Part print with two shaded views. Sizes in mm from the minimum x, y, z corner. Give positions to 0.01 mm unless a question says otherwise; leave off trailing zeros. Write each loop counter-clockwise with the first axis right and the second up, starting at its lowest first coordinate (ties: lowest second). Pieces come first, ordered by that corner, then holes.
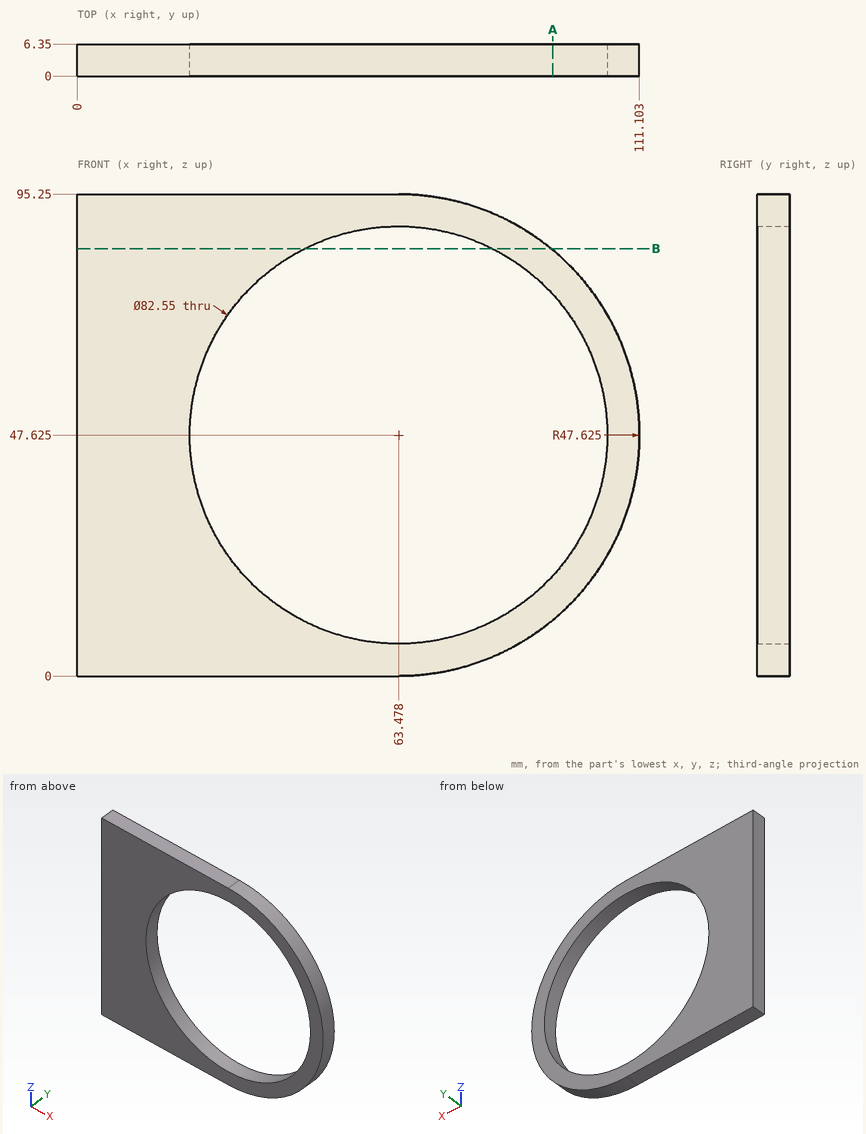
1) Saw through at B-B (z = 84.5). Write the cut outline in (x, y).
Check result:
outline: (0, 0) - (44.93, 0) - (44.93, 6.35) - (0, 6.35) - close; (82.02, 0) - (93.62, 0) - (93.62, 6.35) - (82.02, 6.35) - close
2) Drill centre lines: L1, parallel to X at y = 5.75, z = 46.5; L2, parallel to X at y = 2, z = 69; L3, parallel to Z at x = 46.5, y = 1.5. Where is each one in solid material? Low to high.
Check result:
L1: x = 0 to 22.22, 104.74 to 111.09
L2: x = 0 to 28.17, 98.79 to 106.04
L3: z = 0 to 10, 85.25 to 95.25
3) Flat gauge pins, fed straight in: P1, Ø1, axis at x = 28.5, z = 77, coming from the -Y side; P2, Ø1.5, axis at x = 86, y = 4, coming from the +Z side. Where does each tip first touch, or does it go through?
Check result:
P1: stops at y = 0
P2: stops at z = 89.98
4) Saw through at A-A (x = 94). Write the cut outline in (y, z), and give its area (3 significant figures).
Check result:
outline: (0, 11.07) - (6.35, 11.07) - (6.35, 19.84) - (0, 19.84) - close; (0, 75.41) - (6.35, 75.41) - (6.35, 84.18) - (0, 84.18) - close
area: 111 mm2
